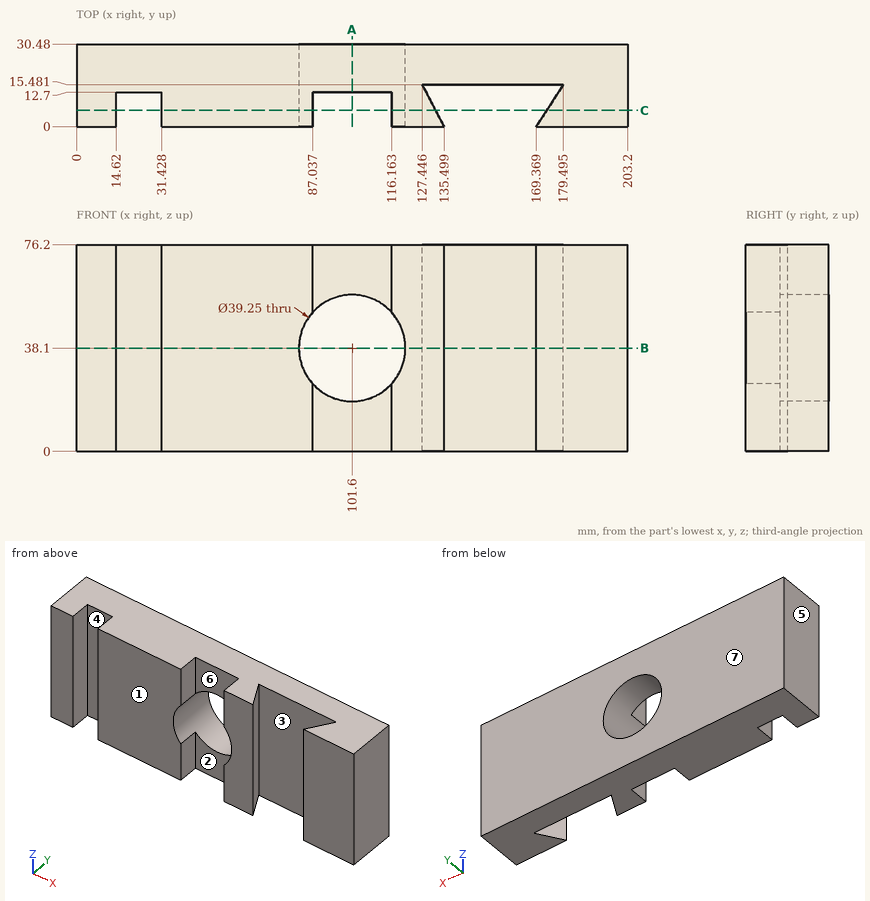
Study the drawing (mm; zero at the part's minimum x, y, z) and answer. A direction names the side the tool comes from. Coordinates: 2 decimals unless noted, no trailing zeros. Write each loop counter-clockwise with the first axis right and the second up, starting at its lowest first coordinate (ties: lowest second). Pieces come first, ordered by that corner, then holes. Notation, with made-up numbers: M 38.5,53 L 86.5,53 A17 cw 86.5,61 Z; hole C 28.25,-3 d5. An arc over 180 degrees is marked long. Use a Markdown table: item, result. Add a question column.
1. Given P1, Ø14, axis at y = 6, z = 60, coming from the -X side; P2, Ø10, axis at x = 149.5, z = 12.5, coming from the -Y side; P3, Ø12.5, axis at x = 100, z = 13, coming from the -Y side, each flat-ended and moving along its own axis, determine where each tip first touches the part or whether it passes through.
2. For a pull along X with two mould halves and no side action, classify the marked faces 4, 5, 6 and 7 as +X half, -X half, draft (parallel to the pull), parting line (faces both ways), or undercut.
3. Section A-A (x = 101.6) is taken. Give the vertices of the cut face in (y, z) (1 decimal).
4. Straight lines are drawn through the part: line 1 along X through (y, z) = (22, 38) (1 decimal); line 2 along Z through (x, y) = (100.5, 22.5) (1 decimal); line 3 along X through (y, z) = (6.5, 72). For each, find the intervals that lie inside material, in ascending order. Write a range as [from, to].
5. Section B-B (z = 38.1) is taken. Give the vertices of the cut face in (x, y) (1 decimal).
6. Which of the six approach directions +Z, -Z, +X, -X, +Y, -Y give full straight-line access (tool end or side, diameter ignored) to the marked faces 1, 2 and 3?
7. Section C-C (y = 6) is taken. Count the separate pieces of the cut face and the enclosed holes in it, plus the area to 3 significant figures.
Data:
| question | item | result |
|---|---|---|
| 1 | P1 | stops at x = 0 |
| 1 | P2 | stops at y = 15.48 |
| 1 | P3 | stops at y = 12.7 |
| 2 | face 4 | undercut |
| 2 | face 5 | -X half |
| 2 | face 6 | undercut |
| 2 | face 7 | draft |
| 3 | outline | M 12.7,0 L 30.5,0 L 30.5,18.5 L 12.7,18.5 Z; M 12.7,57.7 L 30.5,57.7 L 30.5,76.2 L 12.7,76.2 Z |
| 4 | line 1 | x = [0, 82], [121.2, 203.2] |
| 4 | line 2 | z = [0, 18.5], [57.7, 76.2] |
| 4 | line 3 | x = [0, 14.62], [31.43, 87.04], [116.16, 132.12], [173.62, 203.2] |
| 5 | outline | M 0,0 L 14.6,0 L 14.6,12.7 L 31.4,12.7 L 31.4,0 L 82,0 L 82,30.5 L 0,30.5 Z; M 121.2,0 L 135.5,0 L 127.4,15.5 L 179.5,15.5 L 169.4,0 L 203.2,0 L 203.2,30.5 L 121.2,30.5 Z |
| 6 | face 1 | +Z, -Z, +X, -X, -Y |
| 6 | face 2 | +Z, -Z, -Y |
| 6 | face 3 | +Z, -Z |
| 7 | separate pieces | 4 |
| 7 | enclosed holes | 0 |
| 7 | area | 8,680 mm2 |
